```python
from build123d import *

# Parameters (mm, degrees)
BOSS_EXTRUDE1_DEPTH = 3
SKETCH2_R           = 37.5
CUT_EXTRUDE1_DEPTH  = 3
SKETCH3_W           = 4
SKETCH3_H           = 15
BOSS_EXTRUDE4_DEPTH = 3
SKETCH4_W           = 8
SKETCH4_H           = 13
CUT_EXTRUDE2_DEPTH  = 10
CUT_EXTRUDE3_DEPTH  = 10


with BuildPart() as part:
    # Sketch1 → Boss-Extrude1 (new body)
    with BuildSketch(Plane.XY):
        Polygon((11.337032692, 53.818878563), (0, 0), (-220, 0), (-220, 45), (-121.162967308, 73.986910298), align=None)
        Polygon((-94.409209541, 46.483265917), (-94.409209541, 59.799500594), (-120.476048116, 63.767174765), (-179.409209541, 46.483265917), align=None, mode=Mode.SUBTRACT)
    extrude(amount=-BOSS_EXTRUDE1_DEPTH)

    # Sketch2 → Cut-Extrude1 (cut)
    with BuildSketch(Plane.XY):
        with Locations((-182, -15)):
            Circle(SKETCH2_R)
        with Locations((-40, -15)):
            Circle(SKETCH2_R)
    extrude(amount=-CUT_EXTRUDE1_DEPTH, mode=Mode.SUBTRACT)

    # Sketch3 → Boss-Extrude4 (add)
    with BuildSketch(Plane.XY):
        Polygon((-206.731962629, 53.05972607), (-205.606257375, 49.221394704), (-220, 45), (-220, 30), (-224, 30), (-224, 45), (-224, 47.99535863), (-221.125705254, 48.838331367), align=None)
        Polygon((-192.338220004, 57.281120774), (-191.21251475, 53.442789407), (-176.818772125, 57.664184111), (-177.944477379, 61.502515478), align=None)
        Polygon((-121.437734985, 78.074804512), (-106.694649955, 75.830736536), (-107.296563448, 71.876283331), (-121.162967308, 73.986910298), (-133.63754425, 70.328368222), (-134.763249504, 74.166699588), align=None)
        Polygon((-77.03625092, 71.316385344), (-77.638164413, 67.361932139), (-92.46736393, 69.619107735), (-91.865450438, 73.57356094), align=None)
        Polygon((-3.492166825, 56.076054159), (-2.890253333, 60.030507363), (11.938946184, 57.773331767), (16.003099334, 57.297974706), (15.251132951, 52.994367094), (12.159214944, 38.316491123), (8.245114685, 39.141002591), (11.337032692, 53.818878563), align=None)
        Polygon((-18.321366343, 58.333229755), (-17.719452851, 62.287682959), (-32.548652368, 64.544858556), (-33.15056586, 60.590405351), align=None)
        Polygon((-163.550734754, 65.723910181), (-162.4250295, 61.885578815), (-148.031286875, 66.106973518), (-149.156992129, 69.945304885), align=None)
        Polygon((-47.979765378, 62.847580947), (-47.377851886, 66.802034152), (-62.207051403, 69.059209748), (-62.808964895, 65.104756543), align=None)
        with Locations((-222, 7.5)):
            Rectangle(SKETCH3_W, SKETCH3_H)
        Polygon((5.153196678, 24.463126619), (9.067296937, 23.638615151), (5.97537893, 8.960739179), (2.061278671, 9.785250648), align=None)
    extrude(amount=-BOSS_EXTRUDE4_DEPTH)

    # Sketch4 → Cut-Extrude2 (cut)
    with BuildSketch(Plane.XY):
        with Locations((-114.647846568, 25.97260243)):
            Rectangle(SKETCH4_W, SKETCH4_H)
    extrude(amount=-CUT_EXTRUDE2_DEPTH, mode=Mode.SUBTRACT)

    # Sketch5 → Cut-Extrude3 (cut)
    with BuildSketch(Plane.XY):
        with BuildLine():
            Line((-119.647846568, 10.635241704), (-109.647846568, 10.635241704))
            ThreePointArc((-109.647846568, 10.635241704), (-107.647846568, 8.635241704), (-109.647846568, 6.635241704))
            Line((-109.647846568, 6.635241704), (-119.647846568, 6.635241704))
            ThreePointArc((-119.647846568, 6.635241704), (-121.647846568, 8.635241704), (-119.647846568, 10.635241704))
        make_face()
    extrude(amount=-CUT_EXTRUDE3_DEPTH, mode=Mode.SUBTRACT)


solid = part.part
```
Geometry: final body of the model. Coordinates: model frame, mm. A direction names the side the tool comes from. Round coordinates to 2 decimals unless told otherwise and drop trailing zeros. Write each loop counter-clockwise with the first axis right and the second up, starting at its lowest first coordinate (ties: lowest second). Pieces come first, ordered by that corner, then holes.
Item 1: Section query C-C (x = -131.5). Return loops of the section in (y, z), plus the area to 3 significant figures.
Item 2: Mould query, pull axis X, two halves, no side actions, for faces 3 (the face through (-185.04, 59.42, -1.48)), 4 (the face through (-107.26, 61.756, -1.479)), 5 (the face through (-102, 40, 0)). Classes: +X half, -X half, draft (parallel to the pull), parting line (faces both ways), or undercut.
Item 3: Section query D-D (x = -30.5). Return loops of the section in (y, z).
Item 4: Pin query (flat end, axial travel): P1, Ø1.5, axis at y = 28, z = -1, coming from the +X side; P2, Ø1.5, axis at y = 52, z = -2, coming from the +X side; P3, Ø0.9, axis at y = 22.5, z = -2, coming from the -X side. Return the tip coordinate at first contact, or that it passes through.
Item 5: Set-up query: faces 1 (the face through (-149.53, 55.246, -1.479)), 2 (the face through (-102, 40, -3)). Return all of +Z, -Z, +X, -X, +Y, -Y with unobstructed straight access to the full face (end or side cutting, diameter ignored); none if empty.
Item 6: Section query B-B (z = -2.1). Give the number of separate pieces and of enclosed holes in the cut face, plus the area to 3 significant figures.
Item 7: Section query A-A (x = -157). Return loops of the section in (y, z).
Item 8: Material intervals for L1, parallel to Y at x = -94.5, z = -2.1; L2, parallel to X at y = 18, z = -0.05; L3, parallel to X at y = 19, z = -1.35, sorted ascending.
Completed:
1. outline: (0, -3) - (46.48, -3) - (46.48, 0) - (0, 0) - close; (60.53, -3) - (75.12, -3) - (75.12, 0) - (60.53, 0) - close
1. area: 183 mm2
2. face 3: -X half
2. face 4: undercut
2. face 5: draft
3. outline: (21.28, -3) - (64.23, -3) - (64.23, 0) - (21.28, 0) - close
4. P1: stops at x = 6.06
4. P2: stops at x = 15.2
4. P3: stops at x = -220
5. face 1: +Z, -Z
5. face 2: -Z, +X, -X, +Y, -Y
6. separate pieces: 1
6. enclosed holes: 3
6. area: 11,500 mm2
7. outline: (12.95, -3) - (46.48, -3) - (46.48, 0) - (12.95, 0) - close; (53.06, -3) - (67.65, -3) - (67.65, 0) - (53.06, 0) - close
8. L1: y = 0 to 46.48, 59.81 to 69.93
8. L2: x = -220 to -199.81, -164.19 to -57.81, -22.19 to 7.88
8. L3: x = -220 to -197.82, -166.18 to -55.82, -24.18 to 8.09
